The listing builds one solid part. Answer for the finished solid, in the listing's coordinates (mm). A direction names the side the tool comes from. Round coordinates to 2 decimals unless told otherwise and drop trailing zeros. Write each loop counter-clockwise with the first axis right and the second up, starting at its lowest first coordinate (ties: lowest second). Pieces come first, ordered by that corner, then holes. Notation, with made-up numbers: (-37.5, 63.25) -> (-9.5, 63.25) arc R10 cw to (-9.5, 81.25) -> close; hole circle Ø3 at (45, 20.25). An arc over 180 degrees is marked (long way). Write each question's results on one line, items separated by ' | '. Start each with the question number.
```python
from build123d import *

# Parameters (mm, degrees)
F0_W     = 552.45
F0_H     = 304.8
F1_DEPTH = 3.175
F2_W     = 431.8
F2_H     = 152.4
F3_DEPTH = 3.176
F4_R     = 50.8


with BuildPart() as f1:
    # F0 (on Front) → F1 (new body)
    with BuildSketch(Plane.XZ):
        Rectangle(F0_W, F0_H)
    extrude(amount=F1_DEPTH)

    # F2 (on face) → F3 (cut, through all)
    with BuildSketch(Plane.XZ.offset(3.175)):
        with Locations((0, -76.2)):
            Rectangle(F2_W, F2_H)
    extrude(amount=-F3_DEPTH, mode=Mode.SUBTRACT)

    # F4
    f4_edges = [f1.edges().sort_by_distance(p)[0] for p in [
        (-215.9, -1.5875, 0),
        (215.9, -1.5875, 0),
    ]]
    fillet(f4_edges, radius=F4_R)


solid = f1.part
```
Q1. The part is cut by section D-D, the plane x = 83.5. Write down the section's boundary in (y, z) (3 decimals).
Q2. This flat-tipped pin is pushed along its axis until it touches: pin 1 (1.6 mm diameter, centred on x = 37, y = -1, fed in from -Z). Where does it stop, or does it pass through?
Q3. The part is cut by section C-C, the plane z = -83.5. Write down the section's boundary in (x, y) (3 decimals).
Q4. Find the intervals of material crossed by line 1 (X direction, y = -1.9, z = -134.5) (3 decimals); line 2 (Z direction, x = 10, y = -0.4); line 3 (Z direction, x = -183, y = -1.95), in increasing order.
Q5. For faces 1 (the cylindrical face through (-201.414, -1.565, -15.276)), 2 (the flat face through (-4, -3.175, 36)), determine the directions among +Z, -Z, +X, -X, +Y, -Y from which every point of the face is accessible in a straight line to the end or side of a thin tool.
Q6. The part is cut by section A-A, the plane z = -14. Write down the section's boundary in (x, y) (3 decimals), then the cut area to 3 significant figures.
Q7. Determine the mould class of faces 3 (the flat face through (-4, 0, 36)), 4 (the cylindrical face through (201.414, -1.565, -15.276)) for opening direction X: pulls with the +X half, pulls with the -X half, needs draft (parallel to the pull), parting line crosses it, or undercut.
Q8. The part is cut by section B-B, the plane y = -0.7. Write down the section's boundary in (x, z) (3 decimals), then the cut area to 3 significant figures.
Answers follow:
1) outline: (-3.175, 0) -> (0, 0) -> (0, 152.4) -> (-3.175, 152.4) -> close
2) pin 1: z = 0
3) outline: (-276.225, -3.175) -> (-215.9, -3.175) -> (-215.9, 0) -> (-276.225, 0) -> close; (215.9, -3.175) -> (276.225, -3.175) -> (276.225, 0) -> (215.9, 0) -> close
4) line 1: -276.225 to -215.9, 215.9 to 276.225 | line 2: 0 to 152.4 | line 3: -3.26 to 152.4
5) face 1: -Z, +Y, -Y | face 2: +Z, -Z, +X, -X, -Y
6) outline: (-276.225, -3.175) -> (-200.12, -3.175) -> (-200.12, 0) -> (-276.225, 0) -> close; (200.12, -3.175) -> (276.225, -3.175) -> (276.225, 0) -> (200.12, 0) -> close | area: 483 mm^2
7) face 3: needs draft | face 4: undercut
8) outline: (-276.225, -152.4) -> (-215.9, -152.4) -> (-215.9, -50.8) arc R50.8 cw to (-165.1, 0) -> (165.1, 0) arc R50.8 cw to (215.9, -50.8) -> (215.9, -152.4) -> (276.225, -152.4) -> (276.225, 152.4) -> (-276.225, 152.4) -> close | area: 104,000 mm^2
